from build123d import *

# Parameters (mm, degrees)
SKETCH004_W      = 15
SKETCH004_H      = 4
EXTRUDE004_DEPTH = 10
SKETCH001_W      = 119.97
SKETCH001_H      = 73.25
SKETCH001_R      = 1.45
SKETCH001_W_2    = 99.97
SKETCH001_H_2    = 53.25
EXTRUDE001_DEPTH = 22
SKETCH_W         = 99.97
SKETCH_H         = 53.25
EXTRUDE_DEPTH    = 4
FILLET_R         = 5


with BuildPart() as extrude004:
    # Sketch004 (on Face4 of Fusion) → Extrude004 (new body)
    with BuildSketch(Plane(origin=(0, 63.25, 0), x_dir=(-1, 0, 0), z_dir=(0, 1, 0))):
        with Locations((-45.204, 20)):
            Rectangle(SKETCH004_W, SKETCH004_H)
    extrude(amount=-EXTRUDE004_DEPTH)


with BuildPart() as extrude001:
    # Sketch001 (on Sketch) → Extrude001 (new body)
    with BuildSketch(Plane.XY):
        with Locations((49.985, 26.625)):
            Rectangle(SKETCH001_W, SKETCH001_H)
        with Locations((104.97, 58.25)):
            Circle(SKETCH001_R, mode=Mode.SUBTRACT)
        with Locations((104.97, -5)):
            Circle(SKETCH001_R, mode=Mode.SUBTRACT)
        with Locations((-5, -5)):
            Circle(SKETCH001_R, mode=Mode.SUBTRACT)
        with Locations((-5, 58.25)):
            Circle(SKETCH001_R, mode=Mode.SUBTRACT)
        with Locations((49.985, 26.625)):
            Rectangle(SKETCH001_W_2, SKETCH001_H_2, mode=Mode.SUBTRACT)
    extrude(amount=EXTRUDE001_DEPTH)


with BuildPart() as fillet_body:
    # Sketch → Extrude (new body)
    with BuildSketch(Plane.XY):
        with Locations((49.985, 26.625)):
            Rectangle(SKETCH_W, SKETCH_H)
    extrude(amount=EXTRUDE_DEPTH)

    # Fusion: union Extrude001
    add(extrude001.part)

    # Cut001: cut Extrude004
    add(extrude004.part, mode=Mode.SUBTRACT)

    # Fillet
    fillet_edges = [fillet_body.edges().sort_by_distance(p)[0] for p in [
        (-10, 63.25, 11),
        (-10, -10, 11),
        (109.97, 63.25, 11),
        (109.97, -10, 11),
    ]]
    fillet(fillet_edges, radius=FILLET_R)


solid = fillet_body.part
Geometry: final body of the model. Coordinates: model frame, mm. A direction names the side the tool comes from. Coordinates: 2 decimals unless noted, no trailing zeros. Order: outer loops, then holes, each group sorted by start corner. A loop starts at its lowest first (then second) coordinate and runs counter-clockwise, first axis right, second up.
1) Section A-A (x = 27). Return loops of the section in (y, z).
Result sheet:
outline: (-10, 0) - (63.25, 0) - (63.25, 22) - (53.25, 22) - (53.25, 4) - (0, 4) - (0, 22) - (-10, 22) - close
2) Section D-D (z = 19.25). Return loops of the section in (x, y).
Result sheet:
outline: (-10, -5) arc R5 ccw to (-5, -10) - (104.97, -10) arc R5 ccw to (109.97, -5) - (109.97, 58.25) arc R5 ccw to (104.97, 63.25) - (52.7, 63.25) - (52.7, 53.25) - (99.97, 53.25) - (99.97, 0) - (0, 0) - (0, 53.25) - (37.7, 53.25) - (37.7, 63.25) - (-5, 63.25) arc R5 ccw to (-10, 58.25) - close; hole circle Ø2.9 at (-5, -5); hole circle Ø2.9 at (-5, 58.25); hole circle Ø2.9 at (104.97, -5); hole circle Ø2.9 at (104.97, 58.25)
3) Ray query, probe 1 along Y at (x, z) = (-5, 9.25); probe 2 along X at (y, z) = (29.5, 17.5); probe 3 along Y at (x, z) = (2, 7.5). Return the intervals inside material, ascending.
Result sheet:
probe 1: y = -10 to -6.45, -3.55 to 56.8, 59.7 to 63.25
probe 2: x = -10 to 0, 99.97 to 109.97
probe 3: y = -10 to 0, 53.25 to 63.25
4) First-contact query: P1, Ø2.5, axis at x = 104.97, y = -5, coming from the -Z side; P2, Ø3, axis at y = 60, z = 19.5, coming from the -X side; P3, Ø8, axis at x = 42, y = 25, coming from the +Z side. Flat tips, straight axial feed; report the tip coordinate or a pass-through.
Result sheet:
P1: passes through
P2: stops at x = -9.99
P3: stops at z = 4
5) Set-up query: faces 5 (the flat face through (49, 53.25, 13)), 6 (the flat face through (45, 58, 18)), 7 (the cylindrical face through (-5.314, 56.834, 10.846)). Return all of +Z, -Z, +X, -X, +Y, -Y with unobstructed straight access to the full face (end or side cutting, diameter ignored); none if empty.
Result sheet:
face 5: +Z
face 6: +Z, +Y
face 7: +Z, -Z
6) Section B-B (z = 9). Return loops of the section in (x, y).
Result sheet:
outline: (-10, -5) arc R5 ccw to (-5, -10) - (104.97, -10) arc R5 ccw to (109.97, -5) - (109.97, 58.25) arc R5 ccw to (104.97, 63.25) - (-5, 63.25) arc R5 ccw to (-10, 58.25) - close; hole circle Ø2.9 at (-5, -5); hole circle Ø2.9 at (-5, 58.25); hole (0, 0) - (99.97, 0) - (99.97, 53.25) - (0, 53.25) - close; hole circle Ø2.9 at (104.97, -5); hole circle Ø2.9 at (104.97, 58.25)
7) Draft query along Y for faces 1 (the cylindrical face through (108.47, -8.57, 11.15)), 2 (the flat face through (49, 0, 13)), 3 (the flat face through (49, 27, 0)), 4 (the cylindrical face through (106.309, 57.695, 10.846)). Return one class per face: released by +Y, released by -Y, zero draft, split by the parting line, or undercut.
Result sheet:
face 1: released by -Y
face 2: undercut
face 3: zero draft
face 4: undercut
8) Section C-C (y = 35.5). Return loops of the section in (x, z).
Result sheet:
outline: (-10, 0) - (109.97, 0) - (109.97, 22) - (99.97, 22) - (99.97, 4) - (0, 4) - (0, 22) - (-10, 22) - close
